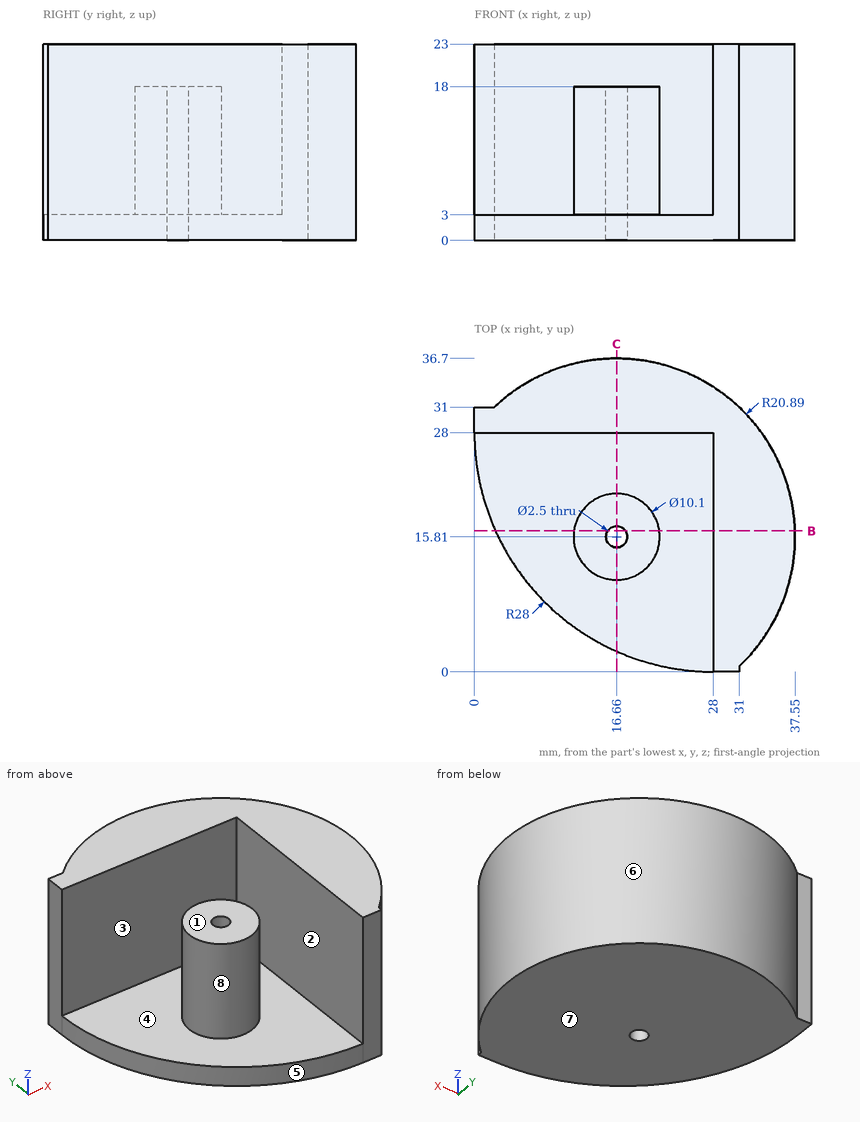
Design review of the part shown in the three views and the two pictorial views. Dimensions are in mm from the part's minimum x, y and z. A direction names the side the tool comes from. Coordinates: 2 decimals unless noted, no trailing zeros. Write each loop counter-clockwise with the first axis right and the second up, starting at its lowest first coordinate (ties: lowest second). Pieces come first, ordered by that corner, then holes.
1) We need section C-C on x = 16.66. State the section outline as (y, z) points.
2) Clearance check with flat-ended pins moving along their axes: pin 1 Ø5 at (y, z) = (31.5, 6) entering from +X; pin 2 Ø2.5 at (x, z) = (1, 7.5) entering from +Y; pin 3 Ø1 at (y, z) = (21, 3) entering from -X (1 decimal); pin 4 Ø10 at (x, y) = (7, 21.5) entering from -Z. State where each tip first meets the part, or that it passes through.
3) The part is to be moulded in two halves that separate along Y. For the marked faces 5, 6, 7 and 8, say which applies: pulls with the +Y half, pulls with the -Y half, needs draft (parallel to the pull), parting line crosses it, or undercut.
4) To check wall thickness, follow probe 1 along Y at (x, z) = (16.66, 6); probe 2 along Z at (x, y) = (23.5, 18); probe 3 along X at (y, z) = (14.5, 11.25). State the ranges of each line that lie inside material, in increasing order.
5) We need section B-B on y = 16.5. State the section outline as (x, z) points.
6) Machinability: for the marked faces 1, 2, 3 and 4, which of the approach directions +Z, -Z, +X, -X, +Y, -Y give a long, thin tool a straight path to every point of the face, cutting with its end or side? Answer none if there is none.
Answer list:
1. outline: (2.4, 0) - (14.56, 0) - (14.56, 18) - (10.76, 18) - (10.76, 3) - (2.4, 3) - close; (17.06, 0) - (36.7, 0) - (36.7, 23) - (28, 23) - (28, 3) - (20.86, 3) - (20.86, 18) - (17.06, 18) - close
2. pin 1: stops at x = 32.86
2. pin 2: stops at y = 31
2. pin 3: stops at x = 0.8
2. pin 4: stops at z = 0
3. face 5: pulls with the -Y half
3. face 6: parting line crosses it
3. face 7: needs draft
3. face 8: undercut
4. probe 1: y = 10.76 to 14.56, 17.06 to 20.86, 28 to 36.7
4. probe 2: z = 0 to 3
4. probe 3: x = 11.78 to 21.54, 28 to 37.51
5. outline: (2.47, 0) - (15.62, 0) - (15.62, 18) - (11.66, 18) - (11.66, 3) - (2.47, 3) - close; (17.7, 0) - (37.54, 0) - (37.54, 23) - (28, 23) - (28, 3) - (21.66, 3) - (21.66, 18) - (17.7, 18) - close
6. face 1: +Z, -X, -Y
6. face 2: +Z, -Y
6. face 3: +Z, -X
6. face 4: +Z
